Check sheet for the modelled part. Datum: model origin and axes. Units: mm. Face numbers are marked on the shaded views. A direction names the side the tool comes from. Coordinates: 2 decimals unless noted, no trailing zeros. Loops run counter-clockwise (first coordinate to the right, second up) from the corner with the lowest first, then second, coordinate; pieces in that order, holes last. Notation, with made-up numbers: M 71.25,-34 L 94.25,-34 A19 ccw 94.25,-20 Z; hole C -40,-11 d10. An arc over 180 degrees is marked long. Answer in a Markdown table with one row per item. Add a question column.
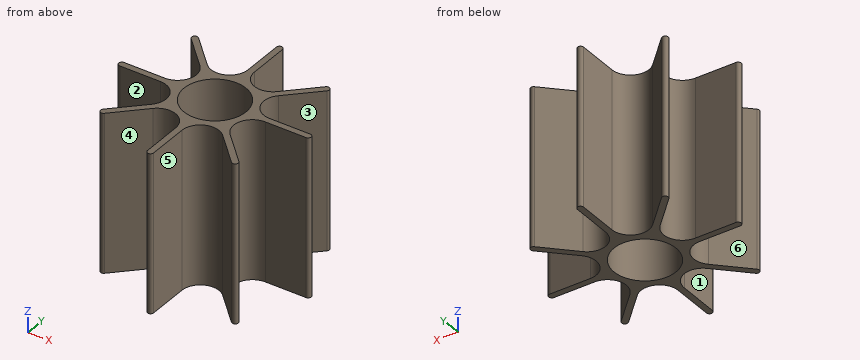
Autodesk Inventor part; units mm, degrees
ref_plane "YZ Plane" through (0, 0, 0) normal (1, 0, 0) x (0, 1, 0)
ref_plane "XZ Plane" through (0, 0, 0) normal (0, 1, 0) x (-1, 0, 0)
ref_plane "XY Plane" through (0, 0, 0) normal (0, 0, 1) x (1, 0, 0)
sketch "Sketch1" plane through (0, 0, 0) normal (0, 0, 1) x (1, 0, 0)
  circle A0 centre (0, 0) radius 5
  circle A1 centre (0, 0) radius 6
  line L0 (5.9791, 0.5) -> (15, 0.5)
  line L1 (5.9791, -0.5) -> (15, -0.5)
  arc A2 (15, -0.5) -> (15, 0.5) centre (15, 0) ccw
  line L2 (0, 0) -> (15, 0) construction
  line L3 (3.8743, 4.5814) -> (10.253, 10.9602)
  arc A3 (10.9602, 10.253) -> (10.253, 10.9602) centre (10.6066, 10.6066) ccw
  line L4 (4.5814, 3.8743) -> (10.9602, 10.253)
  line L5 (-0.5, 5.9791) -> (-0.5, 15)
  arc A4 (0.5, 15) -> (-0.5, 15) centre (0, 15) ccw
  line L6 (0.5, 5.9791) -> (0.5, 15)
  line L7 (-4.5814, 3.8743) -> (-10.9602, 10.253)
  arc A5 (-10.253, 10.9602) -> (-10.9602, 10.253) centre (-10.6066, 10.6066) ccw
  line L8 (-3.8743, 4.5814) -> (-10.253, 10.9602)
  line L9 (-5.9791, -0.5) -> (-15, -0.5)
  arc A6 (-15, 0.5) -> (-15, -0.5) centre (-15, 0) ccw
  line L10 (-5.9791, 0.5) -> (-15, 0.5)
  circle A7 centre (0, 0) radius 15.5 construction
  line L11 (-3.8743, -4.5814) -> (-10.253, -10.9602)
  arc A8 (-10.9602, -10.253) -> (-10.253, -10.9602) centre (-10.6066, -10.6066) ccw
  line L12 (-4.5814, -3.8743) -> (-10.9602, -10.253)
  line L13 (0.5, -5.9791) -> (0.5, -15)
  arc A9 (-0.5, -15) -> (0.5, -15) centre (0, -15) ccw
  line L14 (-0.5, -5.9791) -> (-0.5, -15)
  line L15 (4.5814, -3.8743) -> (10.9602, -10.253)
  arc A10 (10.253, -10.9602) -> (10.9602, -10.253) centre (10.6066, -10.6066) ccw
  line L16 (3.8743, -4.5814) -> (10.253, -10.9602)
  point P0 (-4.5814, 3.8743)
  point P1 (4.5814, 3.8743)
  point P2 (3.8743, 4.5814)
  point P3 (-3.8743, -4.5814)
  point P4 (-4.5814, -3.8743)
  dimension "d0" = 10
  dimension "d1" = 1
  dimension "d2" = 1
  dimension "d5" = 15
  dimension "d8" = 360
  dimension "d13" = 31
extrude "Extrusion1" add sketch "Sketch1" along normal blind 25.5
fillet "Fillet1" radius 3 16 edges at (5.9791, 0.5, 12.75) (4.5814, 3.8743, 12.75) (-0.5, 5.9791, 12.75) (5.9791, -0.5, 12.75) (-5.9791, 0.5, 12.75) (-5.9791, -0.5, 12.75) (-4.5814, 3.8743, 12.75) (-3.8743, 4.5814, 12.75) (0.5, 5.9791, 12.75) (3.8743, 4.5814, 12.75) (-3.8743, -4.5814, 12.75) (-4.5814, -3.8743, 12.75) (-0.5, -5.9791, 12.75) (0.5, -5.9791, 12.75) (3.8743, -4.5814, 12.75) (4.5814, -3.8743, 12.75)
properties part number "Valvula"
Q1. Cross-section at B-B (y = 12). Record the cut outline in (x, z).
Q2. Access from +Z, -Z, +X, -X, +Y, -Y to the whole of each face (thin tool, end or side, straight path). Record for the marked faces 1, 2 and 3.
Q3. Thickness scan on L1, parallel to Y at x = -6, z = 11.25; L2, parallel to Y at x = -8, z = 20.75; L3, parallel to X at y = -9, z = 1.75. Record the ranges inside material, lowest first.
Q4. Go/stop test with flat-tipped pins: pin 1 (1.5 mm diameter, centred on x = -11.5, z = 12, fed in from -Y); pin 2 (7 mm diameter, centred on x = -11.5, z = 12, fed in from +Y); pin 3 (5 mm diameter, centred on y = -2.5, z = 16.5, fed in from -X); pin 4 (1 mm diameter, centred on x = -2.5, y = 3.5, fed in from -Z). Record where each tip stops, or that it passes through.
Q5. Cross-section at A-A (x = 0). Record the cut outline in (y, z), plus the area to 4 significant figures.
Q6. Cross-section at C-C (x = -7.5). Count the separate pieces of the cut face and the enclosed holes in it, plus the area to 3 significant figures.
Q7. Mould release check, pull along Y, two halves, no side actions. Record for the marked faces 4, 5 and 6: released by +Y, released by -Y, zero draft, split by the parting line, or undercut.
Answer key:
| question | item | result |
|---|---|---|
| 1 | outline | M -0.5,0 L 0.5,0 L 0.5,25.5 L -0.5,25.5 Z |
| 2 | face 1 | +Z, -Z, -Y |
| 2 | face 2 | +Z, -Z, -X |
| 2 | face 3 | +Z, -Z, +X |
| 3 | L1 | -6.71 to -5.23, -1.77 to 1.77, 5.23 to 6.71 |
| 3 | L2 | -8.71 to -7.29, -0.53 to 0.53, 7.29 to 8.71 |
| 3 | L3 | -9.71 to -8.29, -0.5 to 0.5, 8.29 to 9.71 |
| 4 | pin 1 | y = -11.09 |
| 4 | pin 2 | y = 11.11 |
| 4 | pin 3 | x = -15.5 |
| 4 | pin 4 | through |
| 5 | outline | M -15.5,0 L -5,0 L -5,25.5 L -15.5,25.5 Z; M 5,0 L 15.5,0 L 15.5,25.5 L 5,25.5 Z |
| 5 | area | 535.5 mm^2 |
| 6 | separate pieces | 3 |
| 6 | enclosed holes | 0 |
| 6 | area | 105 mm^2 |
| 7 | face 4 | released by -Y |
| 7 | face 5 | zero draft |
| 7 | face 6 | undercut |
